Autodesk Fusion 360 part; units mm, degrees
sketch "Skizze1" plane through (0, 0, 0) normal (0, 0, 1) x (1, 0, 0)
  circle A0 centre (0, 0) radius 20
  circle A1 centre (0, 0) radius 17.5
  line L0 (2.55, -1.5) -> (-2.55, -1.5)
  line L1 (-2.55, -1.5) -> (-2.55, 1.5)
  line L2 (-2.55, 1.5) -> (2.55, 1.5)
  line L3 (2.55, 1.5) -> (2.55, -1.5)
  line L4 (2.55, -1.5) -> (-2.55, 1.5) construction
  line L5 (-2.55, -1.5) -> (2.55, 1.5) construction
  line L6 (-1.5, 19.9437) -> (-1.8, 19.9437)
  line L7 (-1.8, 19.9437) -> (-1.8, 17.4072)
  line L8 (-1.8, 17.4072) -> (-1.5, 17.4072)
  line L9 (-1.5, 17.4072) -> (-1.5, 19.9437)
  line L10 (1.5, 19.9437) -> (1.8, 19.9437)
  line L11 (1.8, 19.9437) -> (1.8, 17.4072)
  line L12 (1.8, 17.4072) -> (1.5, 17.4072)
  line L13 (1.5, 17.4072) -> (1.5, 19.9437)
  line L14 (-1.5, -17.4356) -> (-2.5152, -19.8412)
  line L15 (-1.8, -17.4072) -> (-2.8105, -19.8015)
  line L16 (0, 0) -> (0, -21.9932) construction
  line L17 (1.8, -17.4072) -> (2.8105, -19.8015)
  line L18 (1.5, -17.4356) -> (2.5152, -19.8412)
  dimension "d1" = 40
  dimension "d2" = 35
  dimension "d3" = 5.1
  dimension "d4" = 3
  dimension "d14" = 0.3
  dimension "d15" = 1.5
  dimension "d16" = 0.3
  dimension "d17" = 1.5
  dimension "d29" = 0.3
  dimension "d30" = 1.5
extrude "Extrusion1" add sketch "Skizze1" along normal blind 2.5 contours A0 A1 L9 L13 | A0 A1 L11 L17 | A1 L8 L9 L12 L13 | A0 A1 L7 L15 | A0 A1 L14 L18
extrude "Extrusion2" add sketch "Skizze1" along normal blind 7.5 contours A1 L8 L9 L12 L13
extrude "Extrusion3" add sketch "Skizze1" along normal blind 2.5 from surface at 5 contours A0 A1 L9 L13 | A0 A1 L11 L17 | A0 A1 L7 L15 | A0 A1 L14 L18
chamfer "Fase1" distance 0.8 angle 45 8 edges at (0, 1.5, 0) (-2.55, 0, 0) (0, -1.5, 0) (2.55, 0, 0) (-2.55, 0, 7.5) (0, 1.5, 7.5) (2.55, 0, 7.5) (0, -1.5, 7.5)
fillet "Abrundung2" radius 1.5 8 edges at (-19.9935, 0.5086, 7.5) (-19.9935, 0.5086, 0) (0, 20, 0) (0, 20, 7.5) (19.9935, 0.5086, 7.5) (0, -20, 7.5) (0, -20, 0) (19.9935, 0.5086, 0)
chamfer "Fase2" distance 1 angle 45 8 edges at (19.9935, 0.5086, 2.5) (-19.9935, 0.5086, 5) (19.9935, 0.5086, 5) (-19.9935, 0.5086, 2.5) (0, 20, 2.5) (0, 20, 5) (0, -20, 5) (0, -20, 2.5)
equation "d16 = d14"
equation "d17 = d15"
Model file for the job. Use its own axes, mm. A direction names the side the tool comes from. Give positions to 0.01 mm unless a question says otherwise; leave off trailing zeros. Write item = value, one per line. Start each with the question number.
1. Drop flat-ended pins along their axis: P1, Ø5, axis at x = -2, y = 0.5, coming from the -Z side; P2, Ø0.9, axis at y = 0, z = 2.5, coming from the -X side; P3, Ø2, axis at y = -6.5, z = 4.5, coming from the +X side; P4, Ø3, axis at y = 19, z = 0.5, coming from the -X side. Give the stop position or say it passes through.
2. Two-plate mould, pull along Z, no slides. Class faces 1 (the flat face through (1.8, 18, 6)), 2 (the conical face through (0, -19.5, 5.5)): pulls with the +Z half, pulls with the -Z half, needs draft (parallel to the pull), parting line crosses it, or undercut.
3. Which spindle directions (+Z, -Z, +X, -X, +Y, -Y) get a long thin tool onto all of the face, cutting with end or side? Do faces 3 (the flat face through (-18, 0, 2.5)), 4 (the cylindrical face through (0.2, -17.5, 3.5)), 5 (the cylindrical face through (0, 17.5, 3.7)), 6 (the conical face through (19.2, 0, 5.2)). Say none if no direction does.
Taken from the geometry:
q1.P1 = 0
q1.P2 = -19.45
q1.P3 = 18.44
q1.P4 = -9.35
q2.face_1 = needs draft
q2.face_2 = undercut
q3.face_3 = -X
q3.face_4 = none
q3.face_5 = +Y
q3.face_6 = +X
